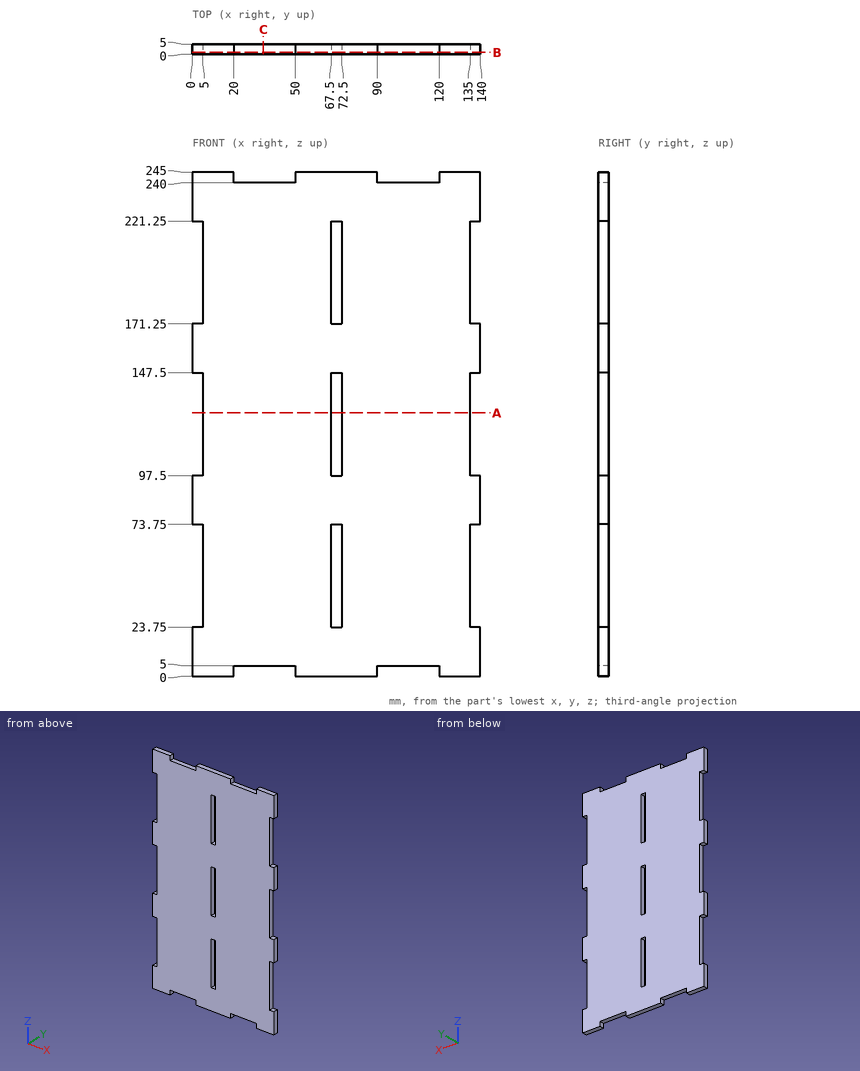
Geometry check sheet. Reference: drawing and pictorial views, mm from the part's lowest x, y, z. Round coordinates to 2 decimals unless told otherwise and drop trailing zeros. Loops run counter-clockwise (first coordinate to the right, second up) from the corner with the lowest first, then second, coordinate; pieces in that order, holes last. Notation, with made-up numbers: (20, 67.5) - (78, 67.5) arc R17 cw to (78, 94.5) - close; hole circle Ø6 at (7.5, 70.25). An arc over 180 degrees is marked (long way). Use a Markdown table: item, result. Add a question column.
1. Section check B-B, the plane y = 0.9. Give the number of separate pieces and of enclosed holes in the cut face, plus the area to 4 significant figures.
2. Thickness scan on probe 1 along X at (y, z) = (0.35, 126.5); probe 2 along Z at (x, y) = (47, 2.5). Record the ranges inside material, lowest first. Write a range as [from, to].
3. Section check C-C, the plane x = 34.5. Record the boundary of the cut face in (y, z).
4. Section check A-A, the plane z = 128. Record the boundary of the cut face in (x, y).
5. Gauge pin test, flat ends, axial feed: pin 1 (2.5 mm diameter, centred on y = 3, z = 53.5, fed in from +X); pin 2 (3 mm diameter, centred on y = 4, z = 199.5, fed in from -X); pin 3 (2.5 mm diameter, centred on x = 38, y = 1.5, fed in from -Z). Record the tip position at first contact, or that the pin passes through.
Checks:
| question | item | result |
|---|---|---|
| 1 | separate pieces | 1 |
| 1 | enclosed holes | 3 |
| 1 | area | 31,450 mm^2 |
| 2 | probe 1 | x = [5, 67.5], [72.5, 135] |
| 2 | probe 2 | z = [5, 240] |
| 3 | outline | (0, 5) - (5, 5) - (5, 240) - (0, 240) - close |
| 4 | outline | (5, 0) - (67.5, 0) - (67.5, 5) - (5, 5) - close; (72.5, 0) - (135, 0) - (135, 5) - (72.5, 5) - close |
| 5 | pin 1 | stops at x = 135 |
| 5 | pin 2 | stops at x = 5 |
| 5 | pin 3 | stops at z = 5 |
